Check sheet for the drawn part. Datum: minimum x, y, z corner. Units: mm. Round coordinates to 2 decimals unless told otherwise and drop trailing zeros. Write each loop counter-clockwise with the first axis right and the second up, starting at its lowest first coordinate (ties: lowest second). Pieces come first, ordered by that corner, then holes. Notation, with made-up numbers: M -21,23.5 L 38,23.5 A35 ccw 38,56.5 Z; hole C 80.25,58.25 d4. An arc over 180 degrees is marked long. Answer in a Markdown table with one row per item. Add a question column.
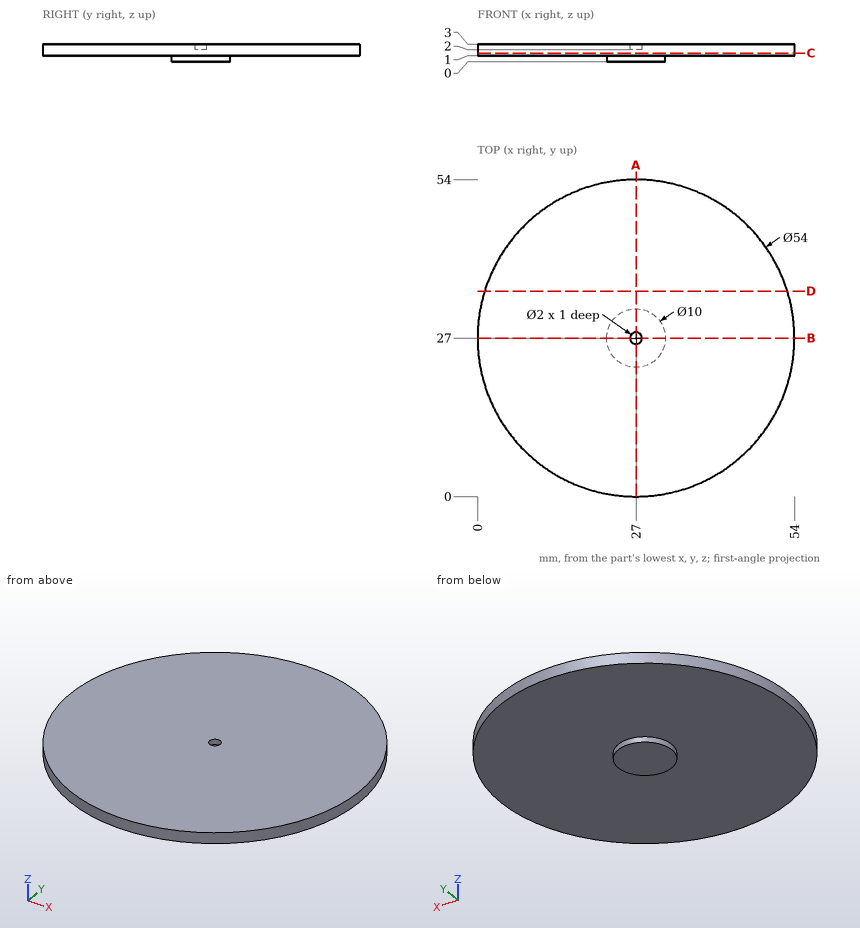
Item 1: Section check D-D, the plane y = 35. Record the boundary of the cut face in (x, z).
Item 2: Gauge pin test, flat ends, axial feed: pin 1 Ø4 at (x, y) = (29.5, 45.5) entering from -Z; pin 2 Ø1.5 at (y, z) = (25.5, 1) entering from -X; pin 3 Ø1.2 at (x, y) = (27, 27) entering from +Z. Record the tip position at first contact, or that the pin passes through.
Item 3: Section check C-C, the plane z = 1.45. Record the boundary of the cut face in (x, y), and give its area (3 significant figures).
Item 4: Section check A-A, the plane x = 27. Record the boundary of the cut face in (y, z), and give its area (3 significant figures).
Item 5: Scan lines: probe 1 along Y at (x, z) = (27, 2.6); probe 2 along Z at (x, y) = (17, 28); probe 3 along X at (y, z) = (31.5, 2.45). Record each from-to range of solid material in increasing order. Write a range as from..to.
Result sheet:
| question | item | result |
|---|---|---|
| 1 | outline | M 1.21,1 L 52.79,1 L 52.79,3 L 1.21,3 Z |
| 2 | pin 1 | stops at z = 1 |
| 2 | pin 2 | stops at x = 0.01 |
| 2 | pin 3 | stops at z = 2 |
| 3 | outline | C 27,27 d54 |
| 3 | area | 2,290 mm^2 |
| 4 | outline | M 0,1 L 22,1 L 22,0 L 32,0 L 32,1 L 54,1 L 54,3 L 28,3 L 28,2 L 26,2 L 26,3 L 0,3 Z |
| 4 | area | 116 mm^2 |
| 5 | probe 1 | y = 0..26, 28..54 |
| 5 | probe 2 | z = 1..3 |
| 5 | probe 3 | x = 0.38..53.62 |
